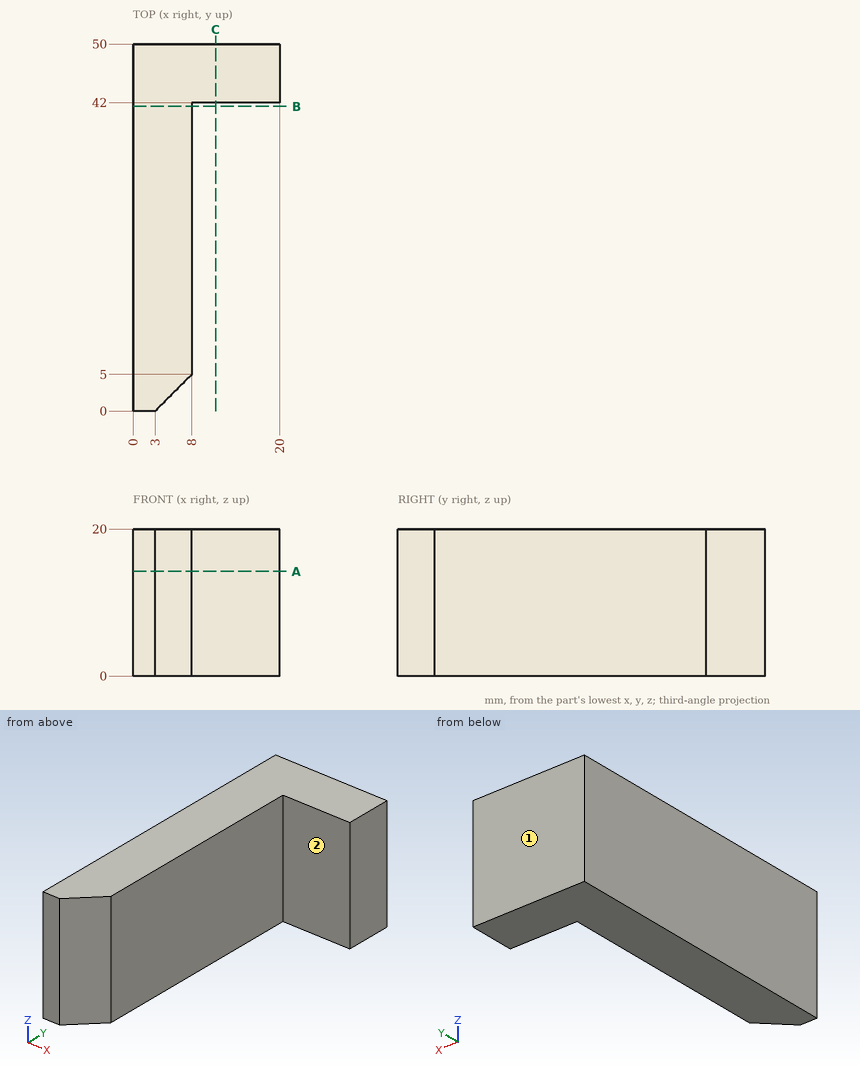
Drawing for the job (mm, zero at the part's lowest x, y, z). A direction names the side the tool comes from. Give positions to 0.01 mm unless a question says otherwise; leave off trailing zeros. Order: outer loops, then holes, each group sorted by start corner. A loop starts at its lowest first (then second) coordinate and runs counter-clockwise, first axis right, second up. Notation, with made-up numbers: (15, 51) -> (34, 51) arc R36 ccw to (34, 90) -> close; hole circle Ø1 at (-13.5, 79.25). An arc over 180 degrees is marked (long way). Use one line per item in the form item = value.
(1) Saw through at C-C (x = 11.25). Write the cut outline in (y, z).
Solution:
outline = (42, 0) -> (50, 0) -> (50, 20) -> (42, 20) -> close
(2) Tool access for the marked faces 1 and 2: list every direction of +Z, -Z, +X, -X, +Y, -Y with a clear straight run to the whole face (end or side of a thin tool).
Solution:
face_1 = +Z, -Z, +X, -X, +Y
face_2 = +Z, -Z, +X, -Y
(3) Flat gauge pins, fed straight in: P1, Ø8, axis at x = 7.5, z = 13.5, coming from the -Y side; P2, Ø1, axis at y = 27.5, z = 6, coming from the +X side; P3, Ø5, axis at x = 12.5, z = 15, coming from the -Y side. Where does each tip first touch, or does it go through?
Solution:
P1 = 0.5
P2 = 8
P3 = 42
(4) Saw through at B-B (y = 41.5). Write the cut outline in (x, z), then the cut area to 3 significant figures.
Solution:
outline = (0, 0) -> (8, 0) -> (8, 20) -> (0, 20) -> close
area = 160 mm²
(5) Saw through at A-A (z = 14.25). Write the cut outline in (x, y).
Solution:
outline = (0, 0) -> (3, 0) -> (8, 5) -> (8, 42) -> (20, 42) -> (20, 50) -> (0, 50) -> close
(6) Drill centre lines: line 1 (Y direction, x = 15.25, z = 9.75); line 2 (X direction, y = 30, z = 10.25); line 3 (Y direction, x = 6.75, z = 8.5). Where is each one in solid material? Low to high. Write a range as from..to.
Solution:
line_1 = 42..50
line_2 = 0..8
line_3 = 3.75..50
